For this review, use the dimensioned drawing (mm, ordinates from the lowest corner) and the shaded views. A direction names the side the tool comes from. Give positions to 0.01 mm unless a question says otherwise; leave off trailing zeros. Loops run counter-clockwise (first coordinate to the right, second up) from the corner with the lowest first, then second, coordinate; pieces in that order, holes last. Notation, with made-up numbers: M -36.75,3.25 L 8.25,3.25 A32 cw 8.25,36.25 Z; hole C 73.5,-21 d11. An arc over 180 degrees is marked long. Use a Markdown table: item, result. Add a question column.
(1) For the marked faces 1, 2 and 3, list the 3-axis set-ups (+Z, -Z, +X, -X, +Y, -Y) from which the entire face can be reached by the end or side of a thin tool; tool diameter is ignored.
(2) Insertion check: pin 1 Ø1.2 at (y, z) = (2, 5) entering from +X; pin 2 Ø0.5 at (y, z) = (2, 5) entering from -X; pin 3 Ø0.5 at (x, y) = (5, 2) entering from -Z. Each pin has a flat end and moves straight along its axis. Give the tip position at first contact, or say it passes through.
(3) Add section B-B, the plane x = 4.75. Give the boundary of the cut face in (y, z), then the cut area to 3 significant figures.
(4) Add section D-D, the plane y = 0.7. Give the boundary of the cut face in (x, z), then the cut area to 3 significant figures.
(5) Add section A-A, the plane z = 4.75. Give the boundary of the cut face in (x, y), then the cut area to 3 significant figures.
(6) For probe 1 along X at (y, z) = (1.35, 7); probe 2 along Y at (x, z) = (4.5, 8), list the stretches that pass through material, from the lowest coordinate up.
(7) Add section C-C, the plane y = 1.7. Give the boundary of the cut face in (x, z).
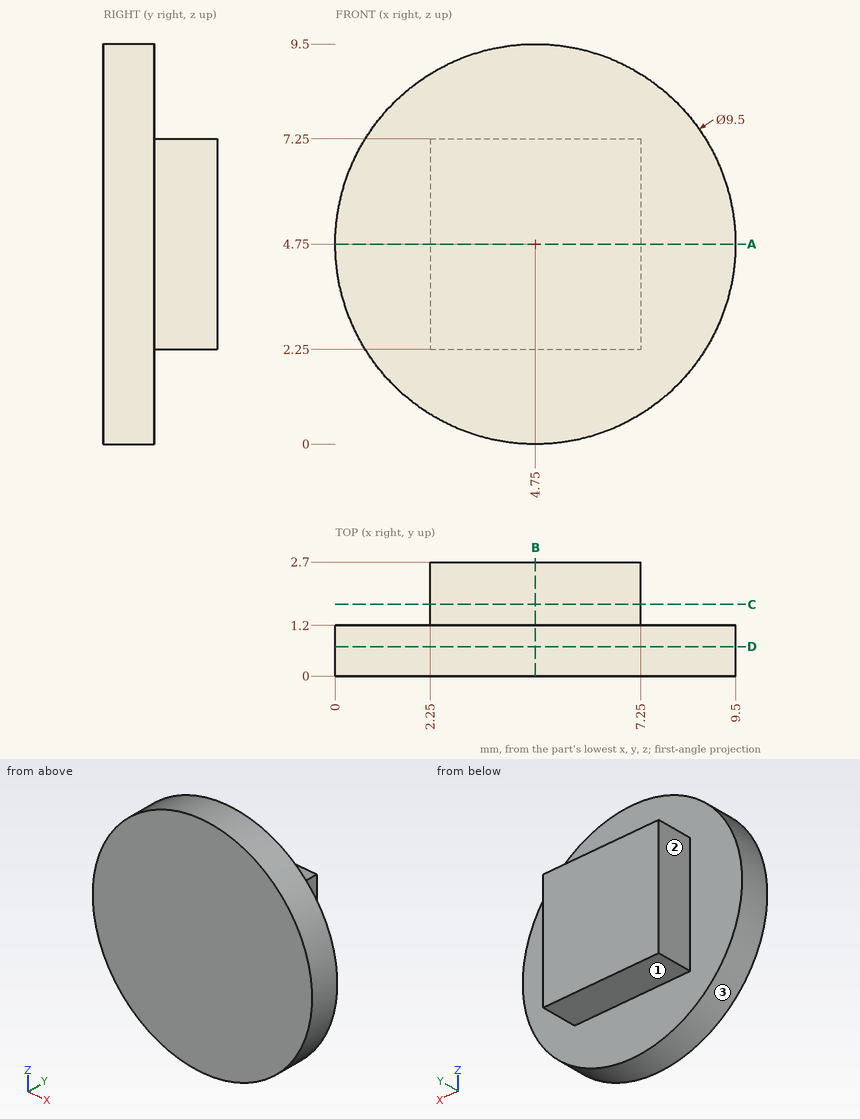
Established:
| question | item | result |
|---|---|---|
| 1 | face 1 | -Z, +X, -X, +Y |
| 1 | face 2 | +Z, -Z, -X, +Y |
| 1 | face 3 | +Y, -Y |
| 2 | pin 1 | x = 7.25 |
| 2 | pin 2 | x = 2.25 |
| 2 | pin 3 | z = 2.25 |
| 3 | outline | M 0,0 L 1.2,0 L 1.2,2.25 L 2.7,2.25 L 2.7,7.25 L 1.2,7.25 L 1.2,9.5 L 0,9.5 Z |
| 3 | area | 18.9 mm^2 |
| 4 | outline | C 4.75,4.75 d9.5 |
| 4 | area | 70.9 mm^2 |
| 5 | outline | M 0,0 L 9.5,0 L 9.5,1.2 L 7.25,1.2 L 7.25,2.7 L 2.25,2.7 L 2.25,1.2 L 0,1.2 Z |
| 5 | area | 18.9 mm^2 |
| 6 | probe 1 | 2.25 to 7.25 |
| 6 | probe 2 | 0 to 1.2 |
| 7 | outline | M 2.25,2.25 L 7.25,2.25 L 7.25,7.25 L 2.25,7.25 Z |
